Read the model definition and answer for the solid it produces. Units are mm, in the model's axes. Face numbers are marked on the shaded views. A direction names the side the tool comes from. Coordinates: 2 decimals unless noted, no trailing zeros. Loops run counter-clockwise (first coordinate to the right, second up) from the corner with the lowest first, then second, coordinate; pieces in that order, holes last. Notation, with made-up numbers: (77, 28) - (99, 28) arc R20 cw to (99, 42) - close; hole circle Ø11 at (-38.75, 85.5). An arc over 180 degrees is marked (long way). Use one line per item in the form item = value. Start each with the question number.
1) A cutting plane is placed at C-C (z = -4.5). Give the vertices of the cut face in (x, y).
2) Consider line 1 (Y direction, x = 1.4, z = -4.5); line 2 (Y direction, x = 2.3, z = 3); line 3 (Z direction, x = 0.55, y = -4.25). Determine where each line is inside the solid, lowest interval first.
3) Which of the six approach directions +Z, -Z, +X, -X, +Y, -Y give full straight-line access (tool end or side, diameter ignored) to the marked faces 1, 2 and 3?
4) A cutting plane is placed at A-A (z = -1). Give the vertices of the cut face in (x, y).
5) The mould has two halves that part along Y. Classify the marked faces 4, 5 and 6: released by +Y, released by -Y, zero draft, split by the parting line, or undercut.
6) A cutting plane is placed at D-D (x = 1.85). Give the vertices of the cut face in (y, z), and give its area (3 significant figures).
7) This flat-tipped pin is pushed along its axis until it touches: P1, Ø5, axis at y = 0, z = -1, coming from the -X side. Where does it stop, or does it pass through?
8) A cutting plane is placed at B-B (y = 0). Give the vertices of the cut face in (x, z).
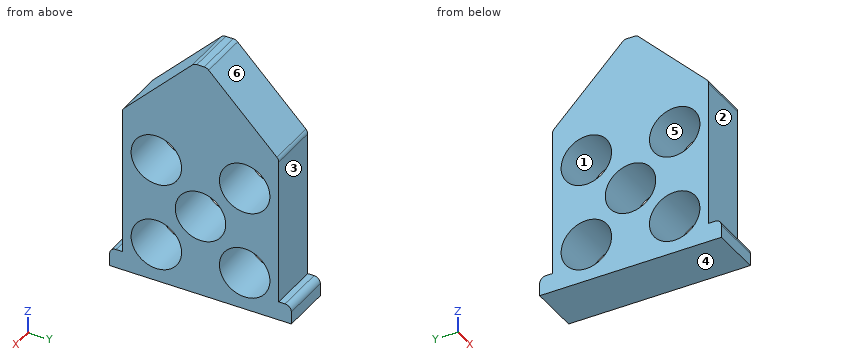
from build123d import *

# Parameters (mm, degrees)
BOSS_EXTRUDE1_DEPTH                = 4
FILLET2_R                          = 0.5
F_4_0MM_MASS_REDUCTION_HOLES_D     = 4
F_4_0MM_MASS_REDUCTION_HOLES_DEPTH = 9.525
F_4_0MM_MASS_REDUCTION_HOLES_TIP   = 1.201721238


with BuildPart() as part:
    # Sketch1 → Boss-Extrude1 (new body)
    with BuildSketch(Plane(origin=(0, 0, 0), x_dir=(0, 0, -1), z_dir=(1, 0, 0))):
        Polygon((-5.8, 6.2), (-11.5, 0.5), (-11.5, -0.5), (-5.8, -6.2), (6, -6.2), (6, -7.2), (7.5, -7.2), (7.5, 7.2), (6, 7.2), (6, 6.2), align=None)
    extrude(amount=BOSS_EXTRUDE1_DEPTH)

    # Fillet2
    fillet2_edges = [part.edges().sort_by_distance(p)[0] for p in [
        (2, -6.2, 5.8),
        (2, -0.5, 11.5),
        (2, 0.5, 11.5),
        (2, 6.2, 5.8),
        (2, 7.2, -6),
        (2, -7.2, -6),
    ]]
    fillet(fillet2_edges, radius=FILLET2_R)

    # Ø4.0mm mass reduction holes
    with Locations(Plane(origin=(4, 0, 0), x_dir=(0, 0, -1), z_dir=(1, 0, 0))):
        with Locations((4.5, -3.5), (4.5, 3.5), (-2.5, -3.5), (-2.5, 3.5), (1, 0)):
            Hole(F_4_0MM_MASS_REDUCTION_HOLES_D / 2, depth=F_4_0MM_MASS_REDUCTION_HOLES_DEPTH)
            with Locations((0, 0, -(F_4_0MM_MASS_REDUCTION_HOLES_DEPTH + F_4_0MM_MASS_REDUCTION_HOLES_TIP / 2))):  # 118° drill point
                Cone(0, F_4_0MM_MASS_REDUCTION_HOLES_D / 2, F_4_0MM_MASS_REDUCTION_HOLES_TIP, mode=Mode.SUBTRACT)


solid = part.part
Found:
q1.outline = (0, -6.2) - (4, -6.2) - (4, -5.5) - (0, -5.5) - close; (0, -1.5) - (4, -1.5) - (4, 1.5) - (0, 1.5) - close; (0, 5.5) - (4, 5.5) - (4, 6.2) - (0, 6.2) - close
q2.line_1 = -6.2 to -5.5, -1.5 to 1.5, 5.5 to 6.2
q2.line_2 = -6.2 to -5.44, -1.56 to 1.56, 5.44 to 6.2
q2.line_3 = -7.5 to -6.35, -2.65 to 0.65, 4.35 to 7.75
q3.face_1 = +X, -X
q3.face_2 = +Z, +X, -X, -Y
q3.face_3 = +Z, +X, -X, +Y
q4.outline = (0, -6.2) - (4, -6.2) - (4, -2) - (0, -2) - close; (0, 2) - (4, 2) - (4, 6.2) - (0, 6.2) - close
q5.face_4 = zero draft
q5.face_5 = undercut
q5.face_6 = released by +Y
q6.outline = (-7.2, -7.5) - (7.2, -7.5) - (7.2, -6.5) arc R0.5 ccw to (6.7, -6) - (6.2, -6) - (6.2, 5.59) arc R0.5 ccw to (6.05, 5.95) - (0.65, 11.35) arc R0.5 ccw to (0.29, 11.5) - (-0.29, 11.5) arc R0.5 ccw to (-0.65, 11.35) - (-6.05, 5.95) arc R0.5 ccw to (-6.2, 5.59) - (-6.2, -6) - (-6.7, -6) arc R0.5 ccw to (-7.2, -6.5) - close; hole circle Ø4 at (-3.5, -4.5); hole circle Ø4 at (-3.5, 2.5); hole circle Ø4 at (0, -1); hole circle Ø4 at (3.5, -4.5); hole circle Ø4 at (3.5, 2.5)
q6.area = 143 mm^2
q7.P1 = 0
q8.outline = (0, -7.5) - (4, -7.5) - (4, -3) - (0, -3) - close; (0, 1) - (4, 1) - (4, 11.5) - (0, 11.5) - close
